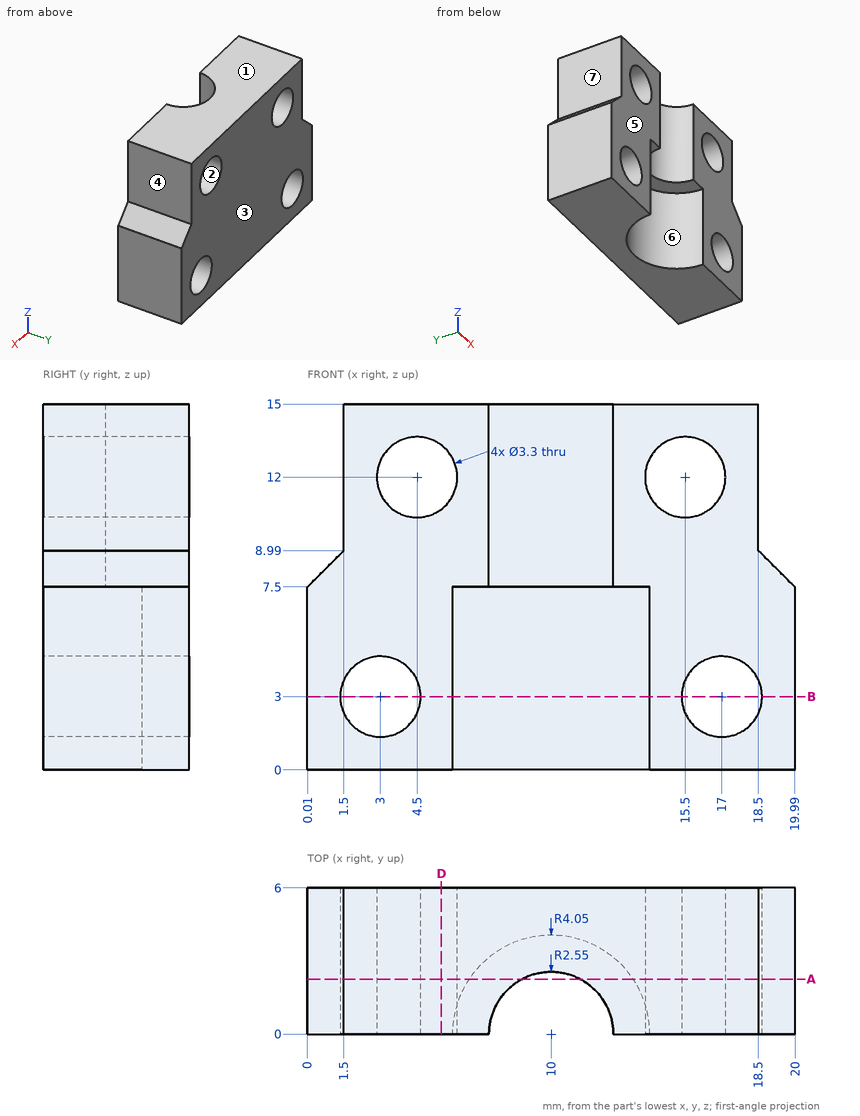
Design review of the part shown in the three views and the two pictorial views. Dimensions are in mm from the part's minimum x, y and z. A direction names the side the tool comes from. Round coordinates to 2 decimals unless told otherwise and drop trailing zeros. Loops run counter-clockwise (first coordinate to the right, second up) from the corner with the lowest first, then second, coordinate; pieces in that order, holes last.
(1) We need section D-D (x = 5.5). Give the boundary of the cut face in (y, z), plus the area to 3 significant figures.
Returned:
outline: (0, 0) - (6, 0) - (6, 10.69) - (0, 10.69) - close; (0, 13.31) - (6, 13.31) - (6, 15) - (0, 15) - close
area: 74.3 mm2
(2) Clearance check with flat-ended pins moving along their axes: P1, Ø3, axis at y = 1.5, z = 9.5, coming from the -X side; P2, Ø1.8, axis at y = 3.5, z = 11.5, coming from the -X side; P3, Ø1.8, axis at y = 3.5, z = 13, coming from the +X side. State where each tip first meets the part, or that it passes through.
Returned:
P1: stops at x = 0.51
P2: stops at x = 1.5
P3: stops at x = 18.5
(3) Mouldability with a two-part tool opening along Z and no side actions: class the marked faces 1, 2 and 3 as released by +Z, released by -Z, zero draft, split by the parting line, or undercut.
Returned:
face 1: released by +Z
face 2: undercut
face 3: zero draft
(4) We need section A-A (y = 2.25). State how many separate pieces and enclosed holes the cut face has, plus the area to 3 significant figures.
Returned:
separate pieces: 2
enclosed holes: 4
area: 177 mm2
(5) We need section B-B (z = 3). Give the boundary of the cut face in (x, y), plus the area to 3 significant figures.
Returned:
outline: (0, 0) - (1.35, 0) - (1.35, 6) - (0, 6) - close; (4.65, 0) - (5.95, 0) arc R4.05 cw to (14.05, 0) - (15.35, 0) - (15.35, 6) - (4.65, 6) - close; (18.65, 0) - (20, 0) - (20, 6) - (18.65, 6) - close
area: 54.6 mm2
(6) Tool access review of the marked faces 4, 5, 6 and 7: name each direction out of +Z, -Z, +X, -X, +Y, -Y from which nothing blocks a thin tool from reaching the whole face with its end or side.
Returned:
face 4: +Z, +X, +Y, -Y
face 5: +Z, -Z, +X, -X, -Y
face 6: -Z, -Y
face 7: +Z, -X, +Y, -Y
(7) Wall thickness on line 1 along X through (y, z) = (3.5, 12.25); line 2 along Z through (x, y) = (4.5, 1.75); line 3 along Z through (x, y) = (4.25, 3.5): over which ranges is each line inside the solid? List them lowest first.
Returned:
line 1: x = 1.5 to 2.87, 6.13 to 13.87, 17.13 to 18.5
line 2: z = 0 to 2.31, 3.69 to 10.35, 13.65 to 15
line 3: z = 0 to 1.92, 4.08 to 10.37, 13.63 to 15
